Part print with two shaded views. Sizes in mm from the minimum x, y, z corner. Coordinates: 2 decimals unless noted, no trailing zeros. Loops run counter-clockwise (first coordinate to the right, second up) from the corner with the lowest first, then second, coordinate; pieces in that order, holes last. Notation, with made-up numbers: (85.25, 49.5) -> (121.25, 49.5) arc R19 cw to (121.25, 65.5) -> close; hole circle Ø3 at (48.25, 41.5). An arc over 180 degrees is marked (long way). Return JSON: item names as keys, results as strings. Group by question number.
(1) Saw through at B-B on z = 4.6. Write the cut outline in (x, y).
(2) Mould opens along Y. For the marked faces 1, 2, 3 and 4 say: pulls with the +Y half, pulls with the -Y half, needs draft (parallel to the pull), parting line crosses it, or undercut.
(3) Saw through at A-A on y = 20. Write the cut outline in (x, z).
(4) Saw through at D-D on x = 15.75. Write the cut outline in (y, z).
(5) Flat gauge pins, fed straight in: pin 1 Ø2 at (y, z) = (26, 2.5) entering from -X; pin 2 Ø3 at (y, z) = (26, 2.5) entering from +X (1 decimal); pin 3 Ø1.5 at (y, z) = (5, 3) entering from -X; pin 4 Ø2 at (y, z) = (4, 2.5) entering from -X. Where does each tip first touch, or does it go through?
(6) Saw through at C-C on y = 4. Write the cut outline in (x, z).
(7) Probe L1, parallel to Y at x = 4.5, z = 2.5; L2, parallel to Z at x = 3.75, y = 26; L3, parallel to Y at x = 6.75, z = 2.5. List the from-to ranges inside material, lowest first.
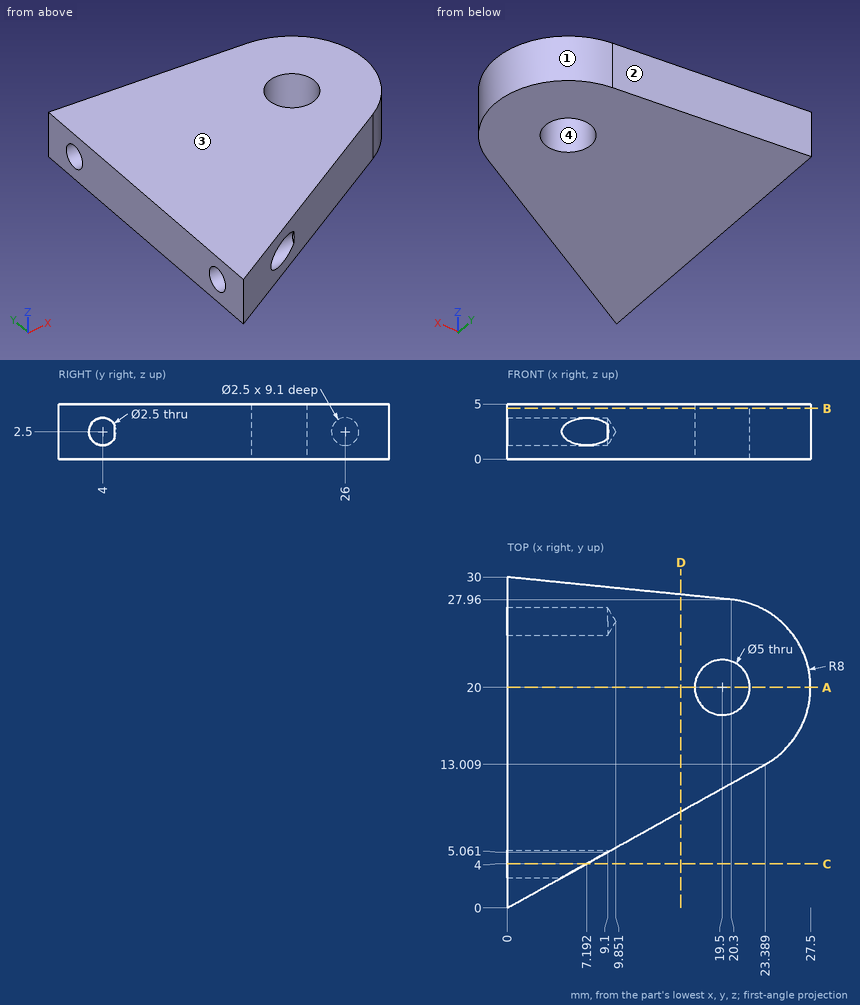
Geometry results:
{
 "1": {"outline": "(0, 0) -> (23.39, 13.01) arc R8 ccw to (20.3, 27.96) -> (0, 30) -> close; hole circle Ø5 at (19.5, 20)"},
 "2": {"face 1": "parting line crosses it", "face 2": "pulls with the +Y half", "face 3": "needs draft", "face 4": "undercut"},
 "3": {"outline": "(0, 0) -> (17, 0) -> (17, 5) -> (0, 5) -> close; (22, 0) -> (27.5, 0) -> (27.5, 5) -> (22, 5) -> close"},
 "4": {"outline": "(8.76, 0) -> (28.42, 0) -> (28.42, 5) -> (8.76, 5) -> close"},
 "5": {"pin 1": "x = 9.25", "pin 2": "x = 26.1", "pin 3": "x = 0", "pin 4": "through"},
 "6": {"outline": "(0, 0) -> (7.19, 0) -> (7.19, 1.25) -> (0, 1.25) -> close; (0, 3.75) -> (7.19, 3.75) -> (7.19, 5) -> (0, 5) -> close"},
 "7": {"L1": "2.5 to 2.75, 5.25 to 24.75, 27.25 to 29.55", "L2": "0 to 1.25, 3.75 to 5", "L3": "5.25 to 24.75, 27.25 to 29.32"}
}
